Autodesk Inventor part; units mm, degrees
ref_plane "YZ Plane" through (0, 0, 0) normal (1, 0, 0) x (0, 1, 0)
ref_plane "XZ Plane" through (0, 0, 0) normal (0, 1, 0) x (-1, 0, 0)
ref_plane "XY Plane" through (0, 0, 0) normal (0, 0, 1) x (1, 0, 0)
sketch "Sketch1" plane through (0, 0, 0) normal (0, 1, 0) x (-1, 0, 0)
  line L0 (-75, 47.5) -> (75, 47.5)
  line L1 (75, 47.5) -> (75, -47.5)
  line L2 (75, -47.5) -> (-75, -47.5)
  line L3 (-75, -47.5) -> (-75, 47.5)
  line L4 (-75, 47.5) -> (75, -47.5) construction
  line L5 (75, 47.5) -> (-75, -47.5) construction
  point P0 (0, 0)
  dimension "d0" = 150
  dimension "d1" = 95
extrude "Extrusion1" add sketch "Sketch1" along normal blind 3
sketch "Sketch6" plane through (0, 3, 0) normal (0, 1, 0) x (1, 0, 0)
  line L0 (75, 47.5) -> (-75, 47.5)
  line L1 (0, 47.5) -> (0, 22.5)
  line L2 (0, 22.5) -> (0, -20.7)
  line L3 (0, -20.7) -> (0, 0.9)
  line L4 (0, 0.9) -> (-53.4, 0.9)
  line L5 (-18.65, 0.9) -> (18.65, 0.9)
  circle A0 centre (18.65, 0.9) radius 2.5
  circle A1 centre (-18.65, 0.9) radius 2.5
  line L6 (-18.65, 0.9) -> (-16.65, 0.9)
  line L7 (18.65, 0.9) -> (16.65, 0.9)
  circle A2 centre (16.65, 0.9) radius 2.5
  circle A3 centre (-16.65, 0.9) radius 2.5
  line L8 (-18.65, 3.4) -> (-16.65, 3.4)
  line L9 (-18.65, -1.6) -> (-16.65, -1.6)
  line L10 (16.65, 3.4) -> (18.65, 3.4)
  line L11 (16.65, -1.6) -> (18.65, -1.6)
  point P0 (0, 0)
  dimension "d40" = 25
  dimension "d41" = 43.2
  dimension "d42" = 53.4
  dimension "d46" = 37.3
  dimension "d47" = 5
  dimension "d48" = 5
  dimension "d49" = 2
  dimension "d50" = 2
  dimension "d51" = 5
  dimension "d52" = 5
extrude "Extrusion6" cut sketch "Sketch6" against normal through all
sketch "Sketch7" plane through (0, 3, 0) normal (0, 1, 0) x (1, 0, 0)
  line L0 (75, 47.5) -> (-75, 47.5)
  line L1 (-75, -47.5) -> (75, -47.5)
  line L2 (75, 47.5) -> (35, 47.5)
  line L3 (35, 47.5) -> (35, -47.5)
  line L4 (35, -47.5) -> (75, -47.5)
  line L5 (75, -47.5) -> (75, 47.5)
  point P0 (0, 0)
  point P1 (75, -47.5)
  dimension "d55" = 40
extrude "Extrusion7" cut sketch "Sketch7" against normal through all
sketch "Sketch8" plane through (0, 3, 0) normal (0, 1, 0) x (1, 0, 0)
  line L0 (-75, -47.5) -> (35, -47.5)
  line L1 (35, 47.5) -> (-75, 47.5)
  line L2 (0, 47.5) -> (0, -42.5)
  circle A0 centre (0, -42.5) radius 13
  line L3 (0, -42.5) -> (-20, -42.5)
  circle A1 centre (-20, -42.5) radius 1.5
  circle A2 centre (-10, -59.8205) radius 1.5
  circle A3 centre (10, -59.8205) radius 1.5
  circle A4 centre (20, -42.5) radius 1.5
  circle A5 centre (10, -25.1795) radius 1.5
  circle A6 centre (-10, -25.1795) radius 1.5
  circle A7 centre (0, -42.5) radius 10
  point P0 (0, 0)
  point P1 (7, 47.5)
  point P2 (-7, 47.5)
  point P3 (-10, -42.5)
  point P4 (-10, -47.5)
  point P5 (10, -42.5)
  point P6 (10, -47.5)
  point P7 (8.6603, -47.5)
  point P8 (-8.6603, -47.5)
  dimension "d60" = 90
  dimension "d62" = 26
  dimension "d63" = 20
  dimension "d64" = 3
  dimension "d67" = 360
  dimension "d69" = 20
sketch "Sketch9" plane through (-75, 0, 47.5) normal (0, 0, 1) x (1, 0, 0)
  line L0 (110, 0) -> (0, 0)
  line L1 (110, 3) -> (110, 0)
  line L2 (0, 0) -> (110, 0)
  line L3 (110, 0) -> (110, 3)
  line L4 (110, 3) -> (0, 3)
  line L5 (0, 3) -> (0, 0)
  point P0 (75, 0)
extrude "Extrusion9" add sketch "Sketch9" along normal blind 20
extrude "Extrusion10" add sketch "Sketch8" along normal blind 94 contours A0 L3 A7 L0 | L0 A7 A0 | A0 L2 A7 L3 | L0 A7 L2 A0
sketch "Sketch10" plane through (0, 3, 42.5) normal (0, 1, 0) x (1, 0, 0)
  circle A0 centre (0, 0) radius 1
  point P0 (0, 42.5)
  dimension "d77" = 2
extrude "Extrusion11" cut sketch "Sketch10" against normal through all
sketch "Sketch11" plane through (0, 0, 0) normal (0, -1, 0) x (1, 0, 0)
  circle A0 centre (0, 42.5) radius 1
  circle A1 centre (0, 42.5) radius 1
  circle A2 centre (0, 42.5) radius 2
  point P0 (0, 0)
  dimension "d80" = 4
extrude "Extrusion12" add sketch "Sketch11" along normal blind 5
thread "Thread1"
fillet "Fillet2" radius 10 4 edges at (35, 1.5, 67.5) (35, 1.5, -47.5) (-75, 1.5, 67.5) (-75, 1.5, -47.5)
properties part number "TopMount"
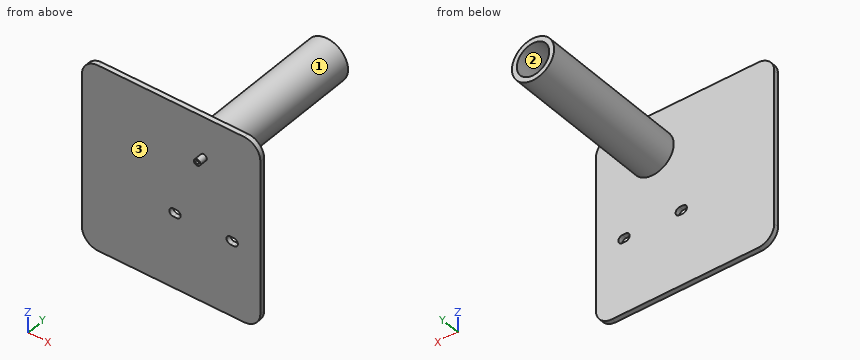
Geometry: final body of the model. Coordinates: model frame, mm. Face numbers are marked on the shaded views. Round coordinates to 2 decimals unless told otherwise and drop trailing zeros. Order: outer loops, then holes, each group sorted by start corner. A loop starts at its lowest first (then second) coordinate and runs counter-clockwise, first axis right, second up. Notation, with made-up numbers: (42, 84.25) -> (64, 84.25) arc R16 cw to (64, 105.25) -> close; hole circle Ø3 at (73, 30). An arc over 180 degrees is marked (long way). Use one line per item in the form item = value. Start each with the question number.
1. Pin query (flat end, axial travel): pin 1 Ø8 at (x, z) = (-27.5, 43) entering from +Y; pin 2 Ø2 at (x, z) = (-31, -31.5) entering from -Y. Return the tip coordinate at first contact, or that it passes through.
2. Cut plane C-C (x = -7). Return the cut outline in (y, z), then the cut area to 3 significant figures.
3. Line query: probe 1 along X at (y, z) = (37, 42); probe 2 along Z at (x, y) = (0, 31); probe 3 along X at (y, z) = (0.25, 42.5). Output: solid intervals per line, ascending.
4. Cut plane A-A (z = -0.9). Return the cut outline in (x, y).
5. Draft query along Z for the marked faces 1, 2 and 3. Return one class per face: pulls with the +Z half, pulls with the -Z half, needs draft (parallel to the pull), parting line crosses it, or undercut.
6. Cut plane B-B (y = 5.5). Return the cut outline in (x, z).
7. Cut plane D-D (z = 22.5). Return the cut outline in (x, y), then the cut area to 3 significant figures.
Solution:
q1.pin_1 = 3
q1.pin_2 = 0
q2.outline = (0, -47.5) -> (3, -47.5) -> (3, 31.55) -> (97, 31.55) -> (97, 35.36) -> (3, 35.36) -> (3, 49.64) -> (97, 49.64) -> (97, 53.45) -> (3, 53.45) -> (3, 67.5) -> (0, 67.5) -> close
q2.area = 1,060 mm^2
q3.probe_1 = -12.99 to -9.99, 9.99 to 12.99
q3.probe_2 = 29.5 to 32.5, 52.5 to 55.5
q3.probe_3 = -75 to -1, 1 to 35
q4.outline = (-75, 0) -> (-21.15, 0) -> (-21.15, 3) -> (-75, 3) -> close; (-14.15, 0) -> (14.15, 0) -> (14.15, 3) -> (-14.15, 3) -> close; (21.15, 0) -> (35, 0) -> (35, 3) -> (21.15, 3) -> close
q5.face_1 = parting line crosses it
q5.face_2 = undercut
q5.face_3 = needs draft
q6.outline = circle Ø26 at (0, 42.5); hole circle Ø20 at (0, 42.5)
q7.outline = (-75, 0) -> (35, 0) -> (35, 3) -> (-75, 3) -> close
q7.area = 330 mm^2
